```python
from build123d import *

# Parameters (mm, degrees)
SKETCH1_W           = 33.8
SKETCH1_H           = 55.5
BOSS_EXTRUDE1_DEPTH = 4
SKETCH3_W           = 4
SKETCH3_H           = 7.5
BOSS_EXTRUDE2_DEPTH = 20
SKETCH4_R           = 1.7
CUT_EXTRUDE1_DEPTH  = 20
SKETCH5_W           = 4
SKETCH5_H           = 20
BOSS_EXTRUDE3_DEPTH = 2
SKETCH6_W           = 4
SKETCH6_H           = 20
BOSS_EXTRUDE4_DEPTH = 2
CHAMFER1_SIZE       = 2
CHAMFER3_SIZE       = 1
SKETCH7_W           = 13.8
SKETCH7_H           = 9
BOSS_EXTRUDE5_DEPTH = 4
CHAMFER4_SIZE       = 1
FILLET1_R           = 5
SKETCH8_R           = 1.7
CUT_EXTRUDE2_DEPTH  = 4


with BuildPart() as part:
    # Sketch1 → Boss-Extrude1 (new body)
    with BuildSketch(Plane(origin=(0, 0, 0), x_dir=(1, 0, 0), z_dir=(0, 1, 0))):
        with Locations((16.9, 27.75)):
            Rectangle(SKETCH1_W, SKETCH1_H)
    extrude(amount=BOSS_EXTRUDE1_DEPTH)

    # Sketch3 → Boss-Extrude2 (add)
    with BuildSketch(Plane(origin=(0, 4, 0), x_dir=(1, 0, 0), z_dir=(0, 1, 0))):
        with Locations((9.5, 3.75)):
            Rectangle(SKETCH3_W, SKETCH3_H)
        with Locations((9.5, 51.75)):
            Rectangle(SKETCH3_W, SKETCH3_H)
    extrude(amount=BOSS_EXTRUDE2_DEPTH)

    # Sketch4 → Cut-Extrude1 (cut)
    with BuildSketch(Plane.ZY.offset(-7.5)):
        with Locations((-3, 19)):
            Circle(SKETCH4_R)
        with Locations((-3, 9)):
            Circle(SKETCH4_R)
        with Locations((-52.5, 9)):
            Circle(SKETCH4_R)
        with Locations((-52.5, 19)):
            Circle(SKETCH4_R)
    extrude(amount=-CUT_EXTRUDE1_DEPTH, mode=Mode.SUBTRACT)

    # Sketch5 → Boss-Extrude3 (add)
    with BuildSketch(Plane.XY):
        with Locations((9.5, 14)):
            Rectangle(SKETCH5_W, SKETCH5_H)
    extrude(amount=BOSS_EXTRUDE3_DEPTH)

    # Sketch6 → Boss-Extrude4 (add)
    with BuildSketch(Plane(origin=(0, 0, -55.5), x_dir=(-1, 0, 0), z_dir=(0, 0, -1))):
        with Locations((-9.5, 14)):
            Rectangle(SKETCH6_W, SKETCH6_H)
    extrude(amount=BOSS_EXTRUDE4_DEPTH)

    # Chamfer1
    chamfer1_edges = [part.edges().sort_by_distance(p)[0] for p in [
        (9.5, 4, 0),
        (9.5, 4, -55.5),
    ]]
    chamfer(chamfer1_edges, length=CHAMFER1_SIZE - 0.0001)  # a hair under: the kernel refuses the full size

    # Chamfer3
    chamfer3_edges = [part.edges().sort_by_distance(p)[0] for p in [
        (9.5, 24, 2),
        (9.5, 24, -57.5),
    ]]
    chamfer(chamfer3_edges, length=CHAMFER3_SIZE)

    # Sketch7 → Boss-Extrude5 (add)
    with BuildSketch(Plane.XZ):
        with Locations((16.9, 4.5)):
            Rectangle(SKETCH7_W, SKETCH7_H)
        with Locations((16.9, -60)):
            Rectangle(SKETCH7_W, SKETCH7_H)
    extrude(amount=-BOSS_EXTRUDE5_DEPTH)

    # Chamfer4
    chamfer4_edges = [part.edges().sort_by_distance(p)[0] for p in [
        (28.8, 4, 0),
        (23.8, 2, 0),
        (10, 1.00005, 0),
        (23.8, 4, 4.5),
        (10, 1.00005, -55.5),
        (23.8, 4, -60),
        (23.8, 2, -55.5),
        (28.8, 4, -55.5),
    ]]
    chamfer(chamfer4_edges, length=CHAMFER4_SIZE)

    # Fillet1
    fillet1_edges = [part.edges().sort_by_distance(p)[0] for p in [
        (10, 2, -64.5),
        (23.8, 1.5, -64.5),
        (10, 2, 9),
        (23.8, 1.5, 9),
    ]]
    fillet(fillet1_edges, radius=FILLET1_R)

    # Sketch8 → Cut-Extrude2 (cut)
    with BuildSketch(Plane(origin=(0, 4, 0), x_dir=(1, 0, 0), z_dir=(0, 1, 0))):
        with Locations(Location((16.9, 58.5, 0), (0, 0, 270))):
            Circle(SKETCH8_R)
        with Locations(Location((16.9, -4, 0), (0, 0, 270))):
            Circle(SKETCH8_R)
    extrude(amount=-CUT_EXTRUDE2_DEPTH, mode=Mode.SUBTRACT)


solid = part.part
```
Geometry check sheet. Reference: the model listing, model coordinates, mm. A direction names the side the tool comes from. Coordinates: 2 decimals unless noted, no trailing zeros. Loops run counter-clockwise (first coordinate to the right, second up) from the corner with the lowest first, then second, coordinate; pieces in that order, holes last.
Item 1: Access from +Z, -Z, +X, -X, +Y, -Y to the whole of each face (thin tool, end or side, straight path). Record for faces 5 (the face through (23.8, 1, -58)), 6 (the face through (9, 14, 2)), 7 (the face through (8.8, 3, -56.5)), 8 (the face through (11.5, 14, -3)).
Item 2: Sectioned sample at C-C, the plane y = 9. Record the boundary of the cut face in (x, z).
Item 3: Sectioned sample at A-A, the plane x = 16.9. Record the boundary of the cut face in (y, z).
Item 4: Release check for a two-part mould opening along Z. For faces 1 (the face through (10, 2, 2)), 2 (the face through (9.47, 19.51, -1.38)), 3 (the face through (9, 14, -48)), 4 (the face through (22.3, 2.03, 7.57)) record: released by +Z, released by -Z, zero draft, split by the parting line, or undercut.
Item 5: Sectioned sample at D-D, the plane z = -3. Record the boundary of the cut face in (x, y).
Item 6: Sectioned sample at B-B, the plane y = 15. Record the boundary of the cut face in (x, z).
Item 7: Go/stop test with flat-tipped pins: pin 1 Ø0.9 at (y, z) = (2, 3) entering from +X; pin 2 Ø17 at (x, z) = (23, -44.5) entering from +Y; pin 3 Ø0.9 at (x, y) = (28.5, 2) entering from -Z; pin 4 Ø2 at (y, z) = (20.5, -10) entering from -X. Record where each tip stops, or that it passes through.
Item 8: Thickness scan on line 1 (Y direction, x = 10.5, z = -52.5); line 2 (X direction, y = 1.95, z = -58.5); line 3 (Y direction, x = 12.5, z = -3). Record the ranges inside material, lowest first.
Check result:
1. face 5: -Z, +X, +Y, -Y
1. face 6: +Z, +X, -X, +Y
1. face 7: -Z, -X, -Y
1. face 8: +Z, -Z, +X, +Y
2. outline: (7.5, -57.5) - (11.5, -57.5) - (11.5, -54.2) - (7.5, -54.2) - close; (7.5, -50.8) - (11.5, -50.8) - (11.5, -48) - (7.5, -48) - close; (7.5, -7.5) - (11.5, -7.5) - (11.5, -4.7) - (7.5, -4.7) - close; (7.5, -1.3) - (11.5, -1.3) - (11.5, 2) - (7.5, 2) - close
3. outline: (0, -64.5) - (4, -64.5) - (4, -60.2) - (0, -60.2) - close; (0, -56.8) - (4, -56.8) - (4, 2.3) - (0, 2.3) - close; (0, 5.7) - (4, 5.7) - (4, 9) - (0, 9) - close
4. face 1: zero draft
4. face 2: undercut
4. face 3: undercut
4. face 4: released by +Z
5. outline: (0, 0) - (33.8, 0) - (33.8, 4) - (11.5, 4) - (11.5, 7.3) - (7.5, 7.3) - (7.5, 4) - (0, 4) - close; (7.5, 10.7) - (11.5, 10.7) - (11.5, 17.3) - (7.5, 17.3) - close; (7.5, 20.7) - (11.5, 20.7) - (11.5, 24) - (7.5, 24) - close
6. outline: (7.5, -57.5) - (11.5, -57.5) - (11.5, -48) - (7.5, -48) - close; (7.5, -7.5) - (11.5, -7.5) - (11.5, 2) - (7.5, 2) - close
7. pin 1: stops at x = 23.8
7. pin 2: stops at y = 4
7. pin 3: stops at z = -55.5
7. pin 4: passes through
8. line 1: y = 0 to 7.3, 10.7 to 17.3, 20.7 to 24
8. line 2: x = 10 to 15.2, 18.6 to 23.8
8. line 3: y = 0 to 4
